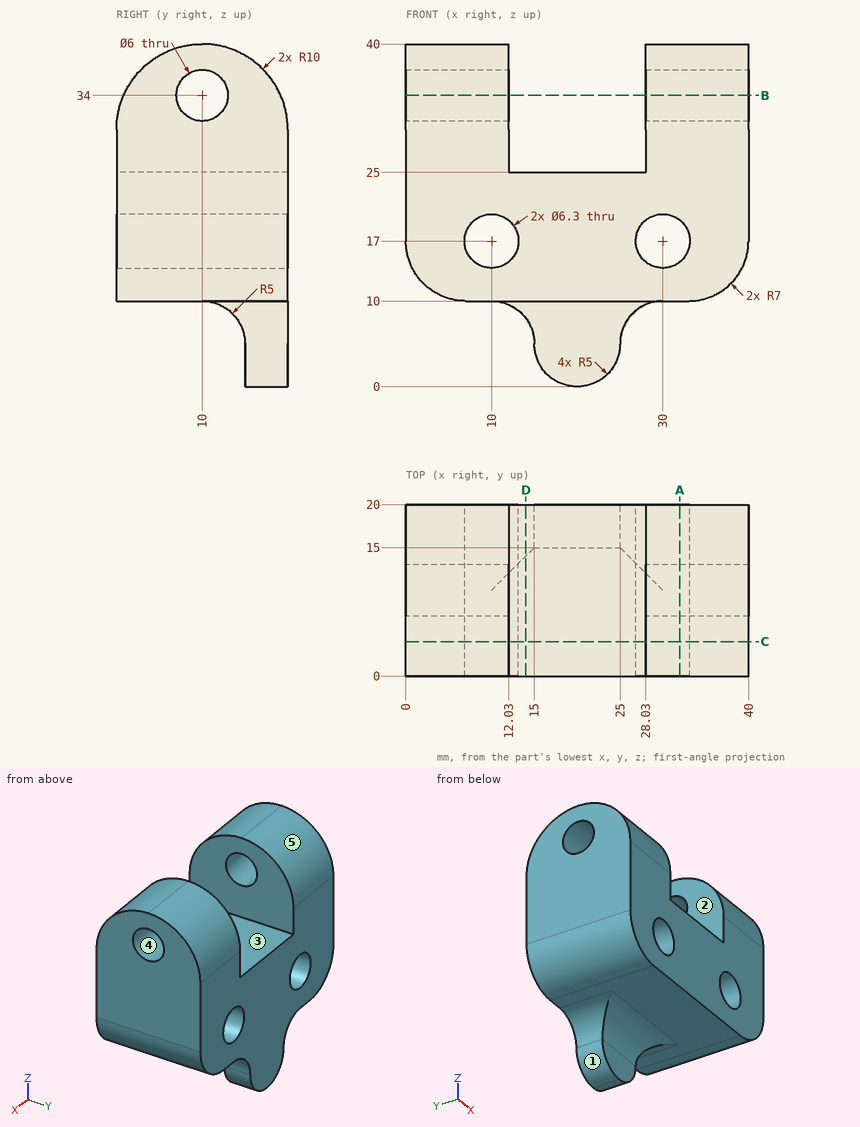
Verification items for this drawing (mm, ordinates from the low corner). A direction names the side the tool comes from. Give positions to 0.01 mm unless a question says otherwise; leave off trailing zeros. Write each loop counter-clockwise with the first axis right and the second up, starting at its lowest first coordinate (ties: lowest second). Pieces come first, ordered by that corner, then holes.
1) Thickness scan on line 1 (X direction, y = 10.25, z = 17); line 2 (Z direction, x = 8, y = 8.5) (1 decimal); line 3 (X direction, y = 17, z = 30). Record the ranges inside material, lowest first.
Values follow:
line 1: x = 0 to 6.85, 13.15 to 26.85, 33.15 to 40
line 2: z = 10 to 14.6, 19.4 to 31.4, 36.6 to 39.9
line 3: x = 0 to 12.03, 28.03 to 40
2) Go/stop test with flat-tipped pins: pin 1 Ø1 at (x, z) = (12.5, 8) entering from +Y; pin 2 Ø1.5 at (x, y) = (34.5, 17.5) entering from -Z; pin 3 Ø2.5 at (x, z) = (20.5, 2) entering from -Y; pin 4 Ø10 at (y, z) = (12, 8) entering from +X (1 decimal). Record where each tip stops, or that it passes through.
Values follow:
pin 1: passes through
pin 2: stops at z = 10.04
pin 3: stops at y = 15
pin 4: stops at x = 38.7
3) Cross-section at A-A (x = 32). Count the separate pieces of the cut face and the enclosed holes in it.
Values follow:
separate pieces: 2
enclosed holes: 1
4) Release check for a two-part mould opening along Y. For the marked faces 3, 4 and 5 record: released by +Y, released by -Y, zero draft, split by the parting line, or undercut.
Values follow:
face 3: zero draft
face 4: undercut
face 5: released by +Y
5) Cross-section at B-B (z = 34). Record the boundary of the cut face in (x, y) (1 decimal), plus the area to 3 significant figures.
Values follow:
outline: (0, 0.8) - (12, 0.8) - (12, 7) - (0, 7) - close; (0, 13) - (12, 13) - (12, 19.2) - (0, 19.2) - close; (28, 0.8) - (40, 0.8) - (40, 7) - (28, 7) - close; (28, 13) - (40, 13) - (40, 19.2) - (28, 19.2) - close
area: 296 mm2
6) Cross-section at D-D (x = 14). Record the boundary of the cut face in (y, z), plus the area to 3 significant figures.
Values follow:
outline: (0, 10) - (10, 10) arc R5 cw to (14, 8) - (20, 8) - (20, 25) - (0, 25) - close
area: 314 mm2
7) Cross-section at C-C (y = 4). Record the boundary of the cut face in (x, z).
Values follow:
outline: (0, 17) arc R7 ccw to (7, 10) - (33, 10) arc R7 ccw to (40, 17) - (40, 38) - (28.03, 38) - (28.03, 25) - (12.03, 25) - (12.03, 38) - (0, 38) - close; hole circle Ø6.3 at (10, 17); hole circle Ø6.3 at (30, 17)
8) Set-up check for the marked faces 1 and 2: record each of +Z, -Z, +X, -X, +Y, -Y from which the full face is reachable in a straight line by a thin tool's end or side.
Values follow:
face 1: -Z, -X, +Y, -Y
face 2: +Z, +Y, -Y
